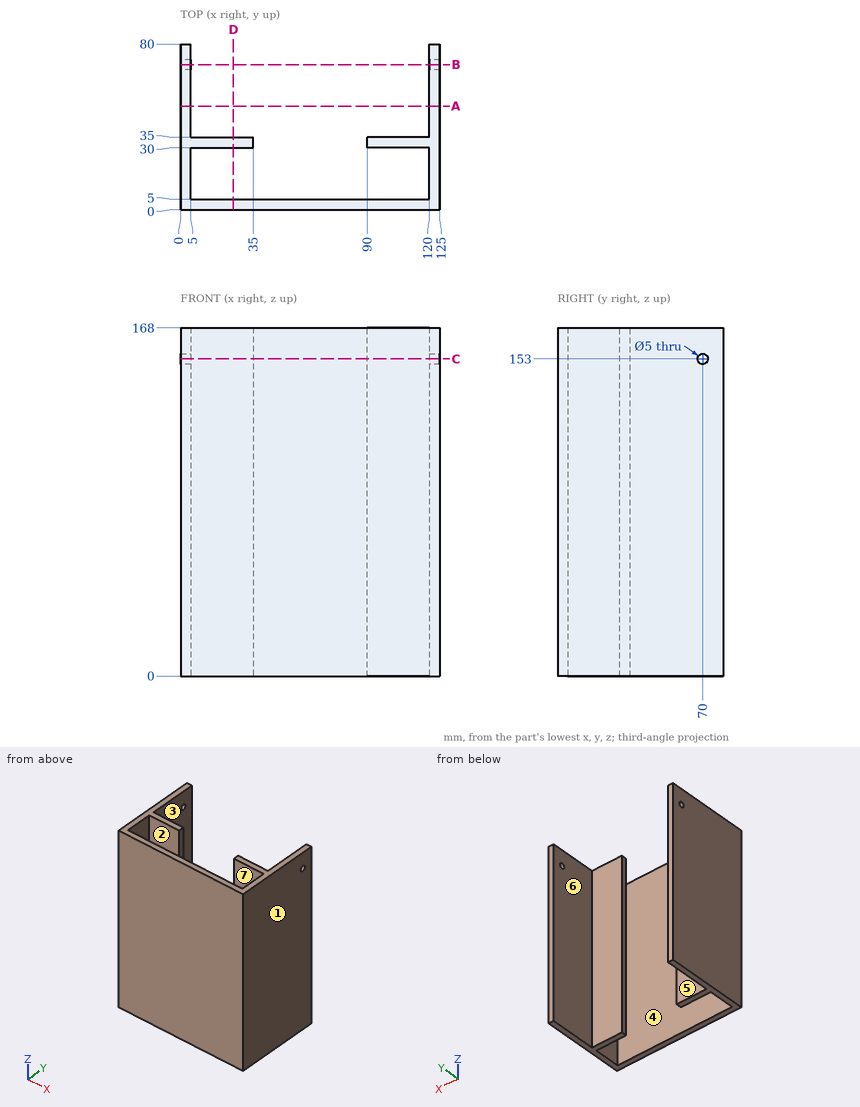
Source: three-view drawing plus pictorial views. Frame: mm from the lowest corner of the part. A direction names the side the tool comes from. Round coordinates to 2 decimals unless told otherwise and drop trailing zeros. Loops run counter-clockwise (first coordinate to the right, second up) from the corner with the lowest first, then second, coordinate; pieces in that order, holes last.
1. Ray query, L1, parallel to X at y = 54.5, z = 120.5; L2, parallel to Y at x = 24, z = 72; L3, parallel to Y at x = 3, z = 153. Return the intervals inside material, ascending.
2. Section query C-C on z = 153. Output: boundary loops of the cut face in (x, y), and give its area (4 significant figures).
3. Contact query for a flat-ended pin moving along its axis: pin 1 (24 mm diameter, centred on x = 99, z = 113.5, fed in from +Y). Output: stop coordinate, or through.
4. Access query for the marked faces 1, 2 and 3. Directions: +Z, -Z, +X, -X, +Y, -Y. A direction counts if a zero-diameter tool reaches every point of the face in a straight line with its end or side. Return the directions, or none.
5. Section query A-A on y = 50. Output: boundary loops of the cut face in (x, z).
6. Mould query, pull axis Y, two halves, no side actions, for the marked faces 4, 5, 6 and 7. Classes: released by +Y, released by -Y, zero draft, split by the parting line, or undercut.
7. Section query D-D on x = 25.5. Output: boundary loops of the cut face in (y, z), and give its area (3 significant figures).
8. Section query B-B on y = 70. Output: boundary loops of the cut face in (x, z), and give its area (3 significant figures).
Answers below:
1. L1: x = 0 to 5, 120 to 125
1. L2: y = 0 to 5, 30 to 35
1. L3: y = 0 to 67.5, 72.5 to 80
2. outline: (0, 0) - (125, 0) - (125, 67.5) - (120, 67.5) - (120, 35) - (90, 35) - (90, 30) - (120, 30) - (120, 5) - (5, 5) - (5, 30) - (35, 30) - (35, 35) - (5, 35) - (5, 67.5) - (0, 67.5) - close; (0, 72.5) - (5, 72.5) - (5, 80) - (0, 80) - close; (120, 72.5) - (125, 72.5) - (125, 80) - (120, 80) - close
2. area: 1,625 mm2
3. pin 1: stops at y = 35
4. face 1: +Z, -Z, +X, +Y, -Y
4. face 2: +Z, -Z
4. face 3: +Z, -Z, +Y
5. outline: (0, 0) - (5, 0) - (5, 168) - (0, 168) - close; (120, 0) - (125, 0) - (125, 168) - (120, 168) - close
6. face 4: undercut
6. face 5: released by +Y
6. face 6: zero draft
6. face 7: undercut
7. outline: (0, 0) - (5, 0) - (5, 168) - (0, 168) - close; (30, 0) - (35, 0) - (35, 168) - (30, 168) - close
7. area: 1,680 mm2
8. outline: (0, 0) - (5, 0) - (5, 150.5) - (0, 150.5) - close; (0, 155.5) - (5, 155.5) - (5, 168) - (0, 168) - close; (120, 0) - (125, 0) - (125, 150.5) - (120, 150.5) - close; (120, 155.5) - (125, 155.5) - (125, 168) - (120, 168) - close
8. area: 1,630 mm2
